from build123d import *

# Parameters (mm, degrees)
F0_R         = 6.35
F1_DEPTH     = 46.9138
F2_R         = 3.048
F3_DEPTH     = 71.12
F4_R         = 3.937
F5_DEPTH     = 12.3698
F6_R         = 6.35
F6_R_2       = 5.6515
F7_DEPTH     = 6.4516
F8_R         = 6.35
F8_R_2       = 4.8514
F9_DEPTH     = 1.524
F10_S5_R     = 3.937
F10_T6_DEPTH = 7
F12_R        = 6.35
F12_R_2      = 5.6134
F13_DEPTH    = 2.159
F15_R        = 6.35
F15_R_2      = 5.6134
F16_DEPTH    = 2.159
F18_R        = 6.35
F18_R_2      = 5.6134
F19_DEPTH    = 2.159
F21_R        = 6.35
F21_R_2      = 5.6134
F22_DEPTH    = 2.159
F24_R        = 6.35
F24_R_2      = 5.6134
F25_DEPTH    = 2.159
F27_R        = 6.35
F27_R_2      = 5.6134
F28_DEPTH    = 2.159
F30_R        = 6.35
F30_R_2      = 5.6134
F31_DEPTH    = 2.159
F33_R        = 6.35
F33_R_2      = 5.6134
F34_DEPTH    = 10.7198
F35_SIZE2    = 5.6134
F35_SIZE     = 4.318


# Not quite as in the source:
# - a fillet or chamfer that OpenCascade refuses, or shapes differently, is made with other operations: its cross-section is extruded or revolved along the edge and cut away or added


with BuildPart() as f1:
    # F0 (on Front) → F1 (new body, symmetric)
    with BuildSketch(Plane.XZ):
        Circle(F0_R)
    extrude(amount=F1_DEPTH, both=True)

    # F2 (on face) → F3 (cut)
    with BuildSketch(Plane.XZ.offset(46.9138)):
        Circle(F2_R)
    extrude(amount=-F3_DEPTH, mode=Mode.SUBTRACT)

    # F4 (on face) → F5 (cut)
    with BuildSketch(Plane.XZ.offset(46.9138)):
        Circle(F4_R)
    extrude(amount=-F5_DEPTH, mode=Mode.SUBTRACT)

    # F6 (on face) → F7 (cut)
    with BuildSketch(Plane.XZ.offset(46.9138)):
        Circle(F6_R)
        Circle(F6_R_2, mode=Mode.SUBTRACT)
    extrude(amount=-F7_DEPTH, mode=Mode.SUBTRACT)

    # F8 (on face) → F9 (cut)
    with BuildSketch(Plane.XZ.offset(40.4622)):
        Circle(F8_R)
        Circle(F8_R_2, mode=Mode.SUBTRACT)
    extrude(amount=-F9_DEPTH, mode=Mode.SUBTRACT)

    # F10: chamfer of 1.016 on 1 edges, made by hand


with BuildPart() as f10_tool2:
    # F10_s3 → F10_t4 (revolve)
    with BuildSketch(Plane.XY):
        Polygon((4.064, -34.544), (3.048, -33.528), (3.048, -34.544), align=None)
    revolve(axis=Axis((0, -34.544, 0), (0, -1, 0)))

    # F10_s5 → F10_t6 (intersect, symmetric)
    with BuildSketch(Plane.XZ.offset(34)):
        Circle(F10_S5_R)
    extrude(amount=F10_T6_DEPTH, both=True, mode=Mode.INTERSECT)


with BuildPart() as f1_1:
    add(f1.part)

    # F10_t1: cut F10_tool2
    add(f10_tool2.part, mode=Mode.SUBTRACT)

    # F12 (on offset) → F13 (cut)
    with BuildSketch(Plane.XZ.offset(34.4678)):
        Circle(F12_R)
        Circle(F12_R_2, mode=Mode.SUBTRACT)
    extrude(amount=-F13_DEPTH, mode=Mode.SUBTRACT)

    # F15 (on offset) → F16 (cut)
    with BuildSketch(Plane.XZ.offset(27.8384)):
        Circle(F15_R)
        Circle(F15_R_2, mode=Mode.SUBTRACT)
    extrude(amount=-F16_DEPTH, mode=Mode.SUBTRACT)

    # F18 (on offset) → F19 (cut)
    with BuildSketch(Plane.XZ.offset(21.209)):
        Circle(F18_R)
        Circle(F18_R_2, mode=Mode.SUBTRACT)
    extrude(amount=-F19_DEPTH, mode=Mode.SUBTRACT)

    # F21 (on offset) → F22 (cut)
    with BuildSketch(Plane.XZ.offset(-4.1402)):
        Circle(F21_R)
        Circle(F21_R_2, mode=Mode.SUBTRACT)
    extrude(amount=-F22_DEPTH, mode=Mode.SUBTRACT)

    # F24 (on offset) → F25 (cut)
    with BuildSketch(Plane.XZ.offset(-10.2616)):
        Circle(F24_R)
        Circle(F24_R_2, mode=Mode.SUBTRACT)
    extrude(amount=-F25_DEPTH, mode=Mode.SUBTRACT)

    # F27 (on offset) → F28 (cut)
    with BuildSketch(Plane.XZ.offset(-21.3868)):
        Circle(F27_R)
        Circle(F27_R_2, mode=Mode.SUBTRACT)
    extrude(amount=-F28_DEPTH, mode=Mode.SUBTRACT)

    # F30 (on offset) → F31 (cut)
    with BuildSketch(Plane.XZ.offset(-28.5496)):
        Circle(F30_R)
        Circle(F30_R_2, mode=Mode.SUBTRACT)
    extrude(amount=-F31_DEPTH, mode=Mode.SUBTRACT)

    # F33 (on offset) → F34 (cut, through all)
    with BuildSketch(Plane.XZ.offset(-36.195)):
        Circle(F33_R)
        Circle(F33_R_2, mode=Mode.SUBTRACT)
    extrude(amount=-F34_DEPTH, mode=Mode.SUBTRACT)

    # F35
    f35_edges = [f1_1.edges().sort_by_distance(p)[0] for p in [
        (-5.6134, 46.9138, 0),
    ]]
    chamfer(f35_edges, length=F35_SIZE, length2=F35_SIZE2)


solid = f1_1.part
Check sheet for the modelled part. Datum: model origin and axes. Units: mm. A direction names the side the tool comes from. Coordinates: 2 decimals unless noted, no trailing zeros. Loops run counter-clockwise (first coordinate to the right, second up) from the corner with the lowest first, then second, coordinate; pieces in that order, holes last. Notation, with made-up numbers: (38.25, -12) -> (67.25, -12) arc R21 cw to (67.25, 8) -> close; hole circle Ø8 at (32, 10). An arc over 180 degrees is marked (long way). Answer in a Markdown table with one row per item.
1. Access from +Z, -Z, +X, -X, +Y, -Y to the whole of each face (thin tool, end or side, straight path). Record for faces 1 (the face through (-1.38, -36.73, -6.2)), 2 (the face through (-0.4, -5.07, 3.02)), 3 (the face through (4.627, -39.711, 1.457)).
Check values:
| item | result |
|---|---|
| face 1 | +Y, -Y |
| face 2 | -Y |
| face 3 | none |
2. Sectioned sample at A-A, the plane y = -20. Record the boundary of the cut face in (x, z).
Check values:
| item | result |
|---|---|
| outline | circle Ø11.23 at (0, 0); hole circle Ø6.1 at (0, 0) |
3. Go/stop test with flat-tipped pins: pin 1 (3 mm diameter, centred on x = -1, z = -0.5, fed in from -Y); pin 2 (4 mm diameter, centred on x = 2, z = -3, fed in from +Y); pin 3 (3.5 mm diameter, centred on x = -1, z = -2, fed in from +Y). Record where each tip stops, or that it passes through.
Check values:
| item | result |
|---|---|
| pin 1 | stops at y = 24.21 |
| pin 2 | stops at y = 45.68 |
| pin 3 | stops at y = 46.54 |
4. Material ranges on line 1 along Z through (x, y) = (0, 12); line 2 along Z through (x, y) = (0, -42.25); line 3 along X through (y, z) = (-18, 2.75), recorded low to high. Write a range as [from, to].
Check values:
| item | result |
|---|---|
| line 1 | z = [-5.61, -3.05], [3.05, 5.61] |
| line 2 | z = [-5.65, -3.94], [3.94, 5.65] |
| line 3 | x = [-5.72, -1.31], [1.31, 5.72] |
5. Release check for a two-part mould opening along X. For faces 4 (the face through (-0.853, -40.753, -3.843)), 5 (the face through (0, 10.262, -6)), 6 (the face through (-1.38, 16.84, -6.2)) record: released by +X, released by -X, zero draft, split by the parting line, or undercut.
Check values:
| item | result |
|---|---|
| face 4 | undercut |
| face 5 | zero draft |
| face 6 | split by the parting line |
